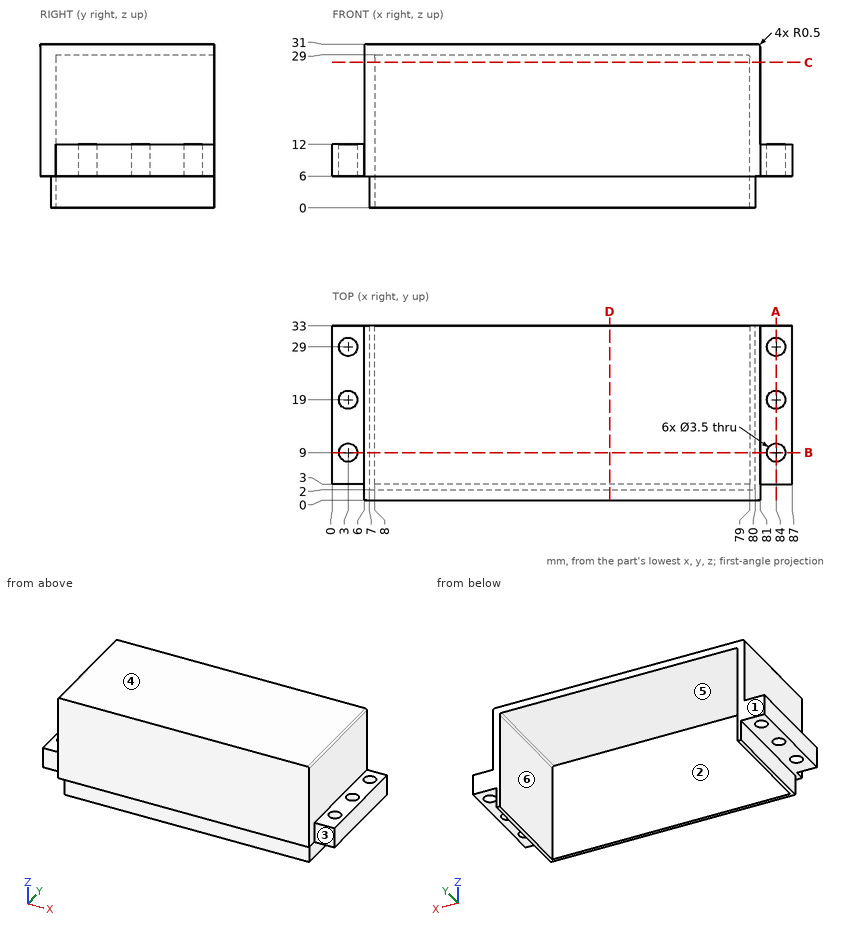
Check sheet for the drawn part. Datum: minimum x, y, z corner. Units: mm. A direction names the side the tool comes from. Give positions to 0.01 mm unless a question says otherwise; leave off trailing zeros. Order: outer loops, then holes, each group sorted by start corner. A loop starts at its lowest first (then second) coordinate and runs counter-clockwise, first axis right, second up. Notation, with made-up numbers: (-4.75, -36.5) - (15.25, -36.5) arc R27 cw to (15.25, 1.5) - close; hole circle Ø4 at (30.5, 84). An arc over 180 degrees is marked (long way). Answer in a Markdown table with one row per item. Add a question column.
Q1. Material ranges on probe 1 along Y at (x, z) = (84, 9); probe 2 along X at (y, z) = (28, 7); probe 3 along X at (y, z) = (16, 17.5), recorded low to high. Write a range as from..to.
Q2. Mould release check, pull along X, two halves, no side actions. Record for the marked faces 4, 5 and 6: pulls with the +X half, pulls with the -X half, needs draft (parallel to the pull), parting line crosses it, or undercut.
Q3. Cross-section at B-B, the plane y = 9. Enter the section's corners in (x, z).
Q4. Cross-section at D-D, the plane x = 52.5. Enter the section's corners in (y, z).
Q5. Gauge pin test, flat ends, axial feed: pin 1 (6.5 mm diameter, centred on x = 84, y = 17, fed in from +Z); pin 2 (1.5 mm diameter, centred on y = 26.5, z = 14, fed in from -X); pin 3 (12 mm diameter, centred on y = 13.5, z = 21.5, fed in from +X); pin 4 (5 mm diameter, centred on y = 16.5, z = 5.5, fed in from +X). Record the tip position at first contact, or that the pin passes through.
Q6. Cross-section at A-A, the plane x = 84. Enter the section's corners in (y, z).
Q7. Tool access check on the marked faces 1, 2 and 3. Record the directions out of +Z, -Z, +X, -X, +Y, -Y that give a thin tool (end or side, any length) a straight path to the whole face; none if there is none.
Q8. Cross-section at C-C, the plane z = 27.5. Enter the section's corners in (x, y), then the cut area to 3 significant figures.
Check values:
| question | item | result |
|---|---|---|
| 1 | probe 1 | y = 3..7.25, 10.75..17.25, 20.75..27.25, 30.75..33 |
| 1 | probe 2 | x = 0..1.56, 4.44..8, 79..82.56, 85.44..87 |
| 1 | probe 3 | x = 6..8, 79..81 |
| 2 | face 4 | needs draft |
| 2 | face 5 | undercut |
| 2 | face 6 | undercut |
| 3 | outline | (0, 6) - (1.25, 6) - (1.25, 12) - (0, 12) - close; (4.75, 6) - (7, 6) - (7, 0) - (8, 0) - (8, 28.5) arc R0.5 cw to (8.5, 29) - (78.5, 29) arc R0.5 cw to (79, 28.5) - (79, 0) - (80, 0) - (80, 6) - (82.25, 6) - (82.25, 12) - (81, 12) - (81, 30.5) arc R0.5 ccw to (80.5, 31) - (6.5, 31) arc R0.5 ccw to (6, 30.5) - (6, 12) - (4.75, 12) - close; (85.75, 6) - (87, 6) - (87, 12) - (85.75, 12) - close |
| 4 | outline | (0, 6) - (2, 6) - (2, 0) - (3, 0) - (3, 29) - (33, 29) - (33, 31) - (0, 31) - close |
| 5 | pin 1 | stops at z = 30.93 |
| 5 | pin 2 | stops at x = 6 |
| 5 | pin 3 | stops at x = 81 |
| 5 | pin 4 | stops at x = 87 |
| 6 | outline | (3, 6) - (7.25, 6) - (7.25, 12) - (3, 12) - close; (10.75, 6) - (17.25, 6) - (17.25, 12) - (10.75, 12) - close; (20.75, 6) - (27.25, 6) - (27.25, 12) - (20.75, 12) - close; (30.75, 6) - (33, 6) - (33, 12) - (30.75, 12) - close |
| 7 | face 1 | +Z, -Z, +X, -X, +Y |
| 7 | face 2 | -Z, +Y |
| 7 | face 3 | +Z, -Z, +X, -Y |
| 8 | outline | (6, 0) - (81, 0) - (81, 33) - (79, 33) - (79, 3) - (8, 3) - (8, 33) - (6, 33) - close |
| 8 | area | 345 mm^2 |
